Could you check a few things on this model? Use its own coordinates, in mm. Face numbers are marked on the shaded views. A direction names the side the tool comes from. Coordinates: 2 decimals unless noted, no trailing zeros. Loops run counter-clockwise (first coordinate to the right, second up) from the corner with the lowest first, then second, coordinate; pieces in that order, holes last. Notation, with made-up numbers: M 54.5,47.25 L 89.5,47.25 A10 cw 89.5,63.25 Z; hole C 49.25,-25 d9. An arc over 180 degrees is marked long. Write each question's results on one line, items separated by ' | '.
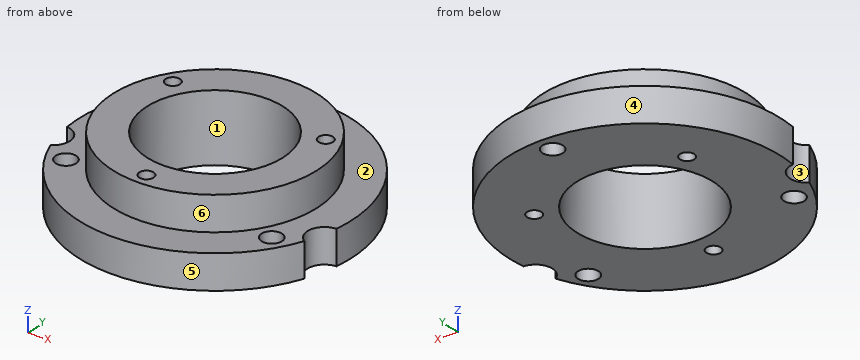
```python
from build123d import *

# Parameters (mm, degrees)
SKETCH_R      = 3
SKETCH_R_2    = 2.1
SKETCH_R_3    = 20
PAD_DEPTH     = 20
SKETCH001_R   = 40
SKETCH001_R_2 = 30
POCKET_DEPTH  = 10


with BuildPart() as part:
    # Sketch → Pad (new body)
    with BuildSketch(Plane.XY):
        with BuildLine():
            ThreePointArc((-37.373806, -14.254775), (0, -40), (37.373806, -14.254775))
            ThreePointArc((39.685017, -5.009931), (35.149287, -8.787322), (37.373806, -14.254775))
            ThreePointArc((39.685017, -5.009931), (0, 40), (-39.685017, -5.009931))
            ThreePointArc((-37.373806, -14.254775), (-35.149287, -8.787322), (-39.685017, -5.009931))
        make_face()
        with Locations((0, 35)):
            Circle(SKETCH_R, mode=Mode.SUBTRACT)
        with Locations((-30.310889, -17.5)):
            Circle(SKETCH_R, mode=Mode.SUBTRACT)
        with Locations((30.310889, -17.5)):
            Circle(SKETCH_R, mode=Mode.SUBTRACT)
        with Locations((-22.51666, 13)):
            Circle(SKETCH_R_2, mode=Mode.SUBTRACT)
        with Locations((22.51666, 13)):
            Circle(SKETCH_R_2, mode=Mode.SUBTRACT)
        with Locations((0, -26)):
            Circle(SKETCH_R_2, mode=Mode.SUBTRACT)
        Circle(SKETCH_R_3, mode=Mode.SUBTRACT)
    extrude(amount=PAD_DEPTH)

    # Sketch001 (on Face13 of Pad) → Pocket (cut)
    with BuildSketch(Plane.XY.offset(20)):
        Circle(SKETCH001_R)
        Circle(SKETCH001_R_2, mode=Mode.SUBTRACT)
    extrude(amount=-POCKET_DEPTH, mode=Mode.SUBTRACT)


solid = part.part
```
(1) If we mould it in two halves opening along X, with no side actions, what happens to the marked faces 1, 2, 3 and 4? For each: released by +X, released by -X, zero draft, split by the parting line, or undercut.
Reported:
face 1: undercut | face 2: zero draft | face 3: released by -X | face 4: split by the parting line
(2) Imagine slicing it at A-A, the plane y = 0. List the corners of the cut face in (x, z) for me.
Reported:
outline: M -40,0 L -20,0 L -20,20 L -30,20 L -30,10 L -40,10 Z; M 20,0 L 40,0 L 40,10 L 30,10 L 30,20 L 20,20 Z
(3) Imagine slicing it at D-D, the plane z = 18. List the corners of the cut face in (x, y) for me.
Reported:
outline: C 0,0 d60; hole C -22.52,13 d4.2; hole C 0,0 d40; hole C 0,-26 d4.2; hole C 22.52,13 d4.2
(4) Will these pins go through, and if not, where does the flat tip stop? P1, Ø4, axis at x = 29, z = 10, coming from the +Y side; P2, Ø8, axis at y = -8, z = 9.5, coming from the +X side; P3, Ø6, axis at x = 7, z = 18, coming from the -Y side.
Reported:
P1: stops at y = 29.51 | P2: stops at x = 39.8 | P3: stops at y = -29.73
(5) Imagine slicing it at C-C, the plane y = 13. List the corners of the cut face in (x, z) for me, and give its area (3 significant figures).
Reported:
outline: M -37.83,0 L -24.62,0 L -24.62,20 L -27.04,20 L -27.04,10 L -37.83,10 Z; M -20.42,0 L -15.2,0 L -15.2,20 L -20.42,20 Z; M 15.2,0 L 20.42,0 L 20.42,20 L 15.2,20 Z; M 24.62,0 L 37.83,0 L 37.83,10 L 27.04,10 L 27.04,20 L 24.62,20 Z | area: 521 mm2
(6) Which directions (+Z, -Z, +X, -X, +Y, -Y) give clear straight access to the entire face, cutting with the end or side of a thin tool? Please do the marked faces 5 and 6.
Reported:
face 5: +Z, -Z, -Y | face 6: +Z
(7) Please list where these lines run through material, in increasing order: probe 1 along Z at (x, y) = (30.5, -4.5); probe 2 along Y at (x, z) = (8.5, 3.5); probe 3 along X at (y, z) = (-27, 3). Write a range as from..to.
Reported:
probe 1: z = 0..10 | probe 2: y = -39.09..-18.1, 18.1..39.09 | probe 3: x = -29.51..-1.85, 1.85..29.51
(8) Imagine slicing it at B-B, the plane x = 8.5. List the corners of the cut face in (y, z) for me.
Reported:
outline: M -39.09,0 L -18.1,0 L -18.1,20 L -28.77,20 L -28.77,10 L -39.09,10 Z; M 18.1,0 L 39.09,0 L 39.09,10 L 28.77,10 L 28.77,20 L 18.1,20 Z
